from build123d import *

# Parameters (mm, degrees)
F0_R     = 1.75
F0_R_2   = 1.981
F0_W     = 100
F0_H     = 7.5
F1_DEPTH = 7.5


with BuildPart() as f1:
    # F0 (on Top) → F1 (new body)
    with BuildSketch(Plane.XY):
        with BuildLine():
            Line((109.467205, 397.377165), (-77.832795, 397.377165))
            ThreePointArc((-77.832795, 397.377165), (-82.322924, 395.517293), (-84.182795, 391.027165))
            Line((-84.182795, 391.027165), (-84.182795, 374.177175))
            Line((-84.182795, 374.177175), (-76.682795, 374.177175))
            Line((-76.682795, 374.177175), (-76.682795, 366.677175))
            Line((-76.682795, 366.677175), (-84.182795, 366.677175))
            Line((-84.182795, 366.677175), (-84.182795, 324.227175))
            Line((-84.182795, 324.227175), (-76.682795, 324.227175))
            Line((-76.682795, 324.227175), (-76.682795, 316.727175))
            Line((-76.682795, 316.727175), (-84.182795, 316.727175))
            Line((-84.182795, 316.727175), (-84.182795, 274.277175))
            Line((-84.182795, 274.277175), (-76.682795, 274.277175))
            Line((-76.682795, 274.277175), (-76.682795, 266.777175))
            Line((-76.682795, 266.777175), (-84.182795, 266.777175))
            Line((-84.182795, 266.777175), (-84.182795, 224.327175))
            Line((-84.182795, 224.327175), (-76.682795, 224.327175))
            Line((-76.682795, 224.327175), (-76.682795, 216.827175))
            Line((-76.682795, 216.827175), (-84.182795, 216.827175))
            Line((-84.182795, 216.827175), (-84.182795, 174.377175))
            Line((-84.182795, 174.377175), (-76.682795, 174.377175))
            Line((-76.682795, 174.377175), (-76.682795, 166.877175))
            Line((-76.682795, 166.877175), (-84.182795, 166.877175))
            Line((-84.182795, 166.877175), (-84.182795, 124.427175))
            Line((-84.182795, 124.427175), (-76.682795, 124.427175))
            Line((-76.682795, 124.427175), (-76.682795, 116.927175))
            Line((-76.682795, 116.927175), (-84.182795, 116.927175))
            Line((-84.182795, 116.927175), (-84.182795, 74.477175))
            Line((-84.182795, 74.477175), (-76.682795, 74.477175))
            Line((-76.682795, 74.477175), (-76.682795, 66.977175))
            Line((-76.682795, 66.977175), (-84.182795, 66.977175))
            Line((-84.182795, 66.977175), (-84.182795, 24.527175))
            Line((-84.182795, 24.527175), (-76.682795, 24.527175))
            Line((-76.682795, 24.527175), (-76.682795, 17.027175))
            Line((-76.682795, 17.027175), (-84.182795, 17.027175))
            Line((-84.182795, 17.027175), (-84.182795, -25.422825))
            Line((-84.182795, -25.422825), (-76.682795, -25.422825))
            Line((-76.682795, -25.422825), (-76.682795, -32.922825))
            Line((-76.682795, -32.922825), (-84.182795, -32.922825))
            Line((-84.182795, -32.922825), (-84.182795, -75.372825))
            Line((-84.182795, -75.372825), (-76.682795, -75.372825))
            Line((-76.682795, -75.372825), (-76.682795, -82.872825))
            Line((-76.682795, -82.872825), (-84.182795, -82.872825))
            Line((-84.182795, -82.872825), (-84.182795, -125.322825))
            Line((-84.182795, -125.322825), (-76.682795, -125.322825))
            Line((-76.682795, -125.322825), (-76.682795, -132.822825))
            Line((-76.682795, -132.822825), (-84.182795, -132.822825))
            Line((-84.182795, -132.822825), (-84.182795, -175.272825))
            Line((-84.182795, -175.272825), (-76.682795, -175.272825))
            Line((-76.682795, -175.272825), (-76.682795, -182.772825))
            Line((-76.682795, -182.772825), (-84.182795, -182.772825))
            Line((-84.182795, -182.772825), (-84.182795, -225.222825))
            Line((-84.182795, -225.222825), (-76.682795, -225.222825))
            Line((-76.682795, -225.222825), (-76.682795, -232.722825))
            Line((-76.682795, -232.722825), (-84.182795, -232.722825))
            Line((-84.182795, -232.722825), (-84.182795, -275.172825))
            Line((-84.182795, -275.172825), (-76.682795, -275.172825))
            Line((-76.682795, -275.172825), (-76.682795, -282.672825))
            Line((-76.682795, -282.672825), (-84.182795, -282.672825))
            Line((-84.182795, -282.672825), (-84.182795, -325.122825))
            Line((-84.182795, -325.122825), (-76.682795, -325.122825))
            Line((-76.682795, -325.122825), (-76.682795, -332.622825))
            Line((-76.682795, -332.622825), (-84.182795, -332.622825))
            Line((-84.182795, -332.622825), (-84.182795, -346.272835))
            ThreePointArc((-84.182795, -346.272835), (-82.322924, -350.762964), (-77.832795, -352.622835))
            Line((-77.832795, -352.622835), (109.467205, -352.622835))
            ThreePointArc((109.467205, -352.622835), (113.957333, -350.762964), (115.817205, -346.272835))
            Line((115.817205, -346.272835), (115.817205, -332.622835))
            Line((115.817205, -332.622835), (108.317205, -332.622835))
            Line((108.317205, -332.622835), (108.317205, -325.122835))
            Line((108.317205, -325.122835), (115.817205, -325.122835))
            Line((115.817205, -325.122835), (115.817205, -282.672835))
            Line((115.817205, -282.672835), (108.317205, -282.672835))
            Line((108.317205, -282.672835), (108.317205, -275.172835))
            Line((108.317205, -275.172835), (115.817205, -275.172835))
            Line((115.817205, -275.172835), (115.817205, -232.722835))
            Line((115.817205, -232.722835), (108.317205, -232.722835))
            Line((108.317205, -232.722835), (108.317205, -225.222835))
            Line((108.317205, -225.222835), (115.817205, -225.222835))
            Line((115.817205, -225.222835), (115.817205, -182.772835))
            Line((115.817205, -182.772835), (108.317205, -182.772835))
            Line((108.317205, -182.772835), (108.317205, -175.272835))
            Line((108.317205, -175.272835), (115.817205, -175.272835))
            Line((115.817205, -175.272835), (115.817205, -132.822835))
            Line((115.817205, -132.822835), (108.317205, -132.822835))
            Line((108.317205, -132.822835), (108.317205, -125.322835))
            Line((108.317205, -125.322835), (115.817205, -125.322835))
            Line((115.817205, -125.322835), (115.817205, -82.872835))
            Line((115.817205, -82.872835), (108.317205, -82.872835))
            Line((108.317205, -82.872835), (108.317205, -75.372835))
            Line((108.317205, -75.372835), (115.817205, -75.372835))
            Line((115.817205, -75.372835), (115.817205, -32.922835))
            Line((115.817205, -32.922835), (108.317205, -32.922835))
            Line((108.317205, -32.922835), (108.317205, -25.422835))
            Line((108.317205, -25.422835), (115.817205, -25.422835))
            Line((115.817205, -25.422835), (115.817205, 17.027165))
            Line((115.817205, 17.027165), (108.317205, 17.027165))
            Line((108.317205, 17.027165), (108.317205, 24.527165))
            Line((108.317205, 24.527165), (115.817205, 24.527165))
            Line((115.817205, 24.527165), (115.817205, 66.977165))
            Line((115.817205, 66.977165), (108.317205, 66.977165))
            Line((108.317205, 66.977165), (108.317205, 74.477165))
            Line((108.317205, 74.477165), (115.817205, 74.477165))
            Line((115.817205, 74.477165), (115.817205, 116.927165))
            Line((115.817205, 116.927165), (108.317205, 116.927165))
            Line((108.317205, 116.927165), (108.317205, 124.427165))
            Line((108.317205, 124.427165), (115.817205, 124.427165))
            Line((115.817205, 124.427165), (115.817205, 166.877165))
            Line((115.817205, 166.877165), (108.317205, 166.877165))
            Line((108.317205, 166.877165), (108.317205, 174.377165))
            Line((108.317205, 174.377165), (115.817205, 174.377165))
            Line((115.817205, 174.377165), (115.817205, 216.827165))
            Line((115.817205, 216.827165), (108.317205, 216.827165))
            Line((108.317205, 216.827165), (108.317205, 224.327165))
            Line((108.317205, 224.327165), (115.817205, 224.327165))
            Line((115.817205, 224.327165), (115.817205, 266.777165))
            Line((115.817205, 266.777165), (108.317205, 266.777165))
            Line((108.317205, 266.777165), (108.317205, 274.277165))
            Line((108.317205, 274.277165), (115.817205, 274.277165))
            Line((115.817205, 274.277165), (115.817205, 316.727165))
            Line((115.817205, 316.727165), (108.317205, 316.727165))
            Line((108.317205, 316.727165), (108.317205, 324.227165))
            Line((108.317205, 324.227165), (115.817205, 324.227165))
            Line((115.817205, 324.227165), (115.817205, 366.677165))
            Line((115.817205, 366.677165), (108.317205, 366.677165))
            Line((108.317205, 366.677165), (108.317205, 374.177165))
            Line((108.317205, 374.177165), (115.817205, 374.177165))
            Line((115.817205, 374.177165), (115.817205, 391.027165))
            ThreePointArc((115.817205, 391.027165), (113.957333, 395.517293), (109.467205, 397.377165))
        make_face()
        with Locations((-59.182573, -285.634338)):
            Circle(F0_R, mode=Mode.SUBTRACT)
        Polygon((-48.162773, -168.857838), (-41.787373, -168.857838), (-29.747773, -168.857838), (-23.372373, -168.857838), (-17.352573, -168.857838), (-17.352573, -180.237038), (-17.352573, -282.395838), (-14.177573, -282.395838), (-14.177573, -284.935838), (-14.177573, -286.586838), (-14.177573, -288.009238), (-13.177573, -288.009238), (-13.177573, -288.872838), (-13.177573, -289.372838), (-14.177573, -289.372838), (-32.592573, -289.372838), (-33.227573, -289.372838), (-51.642573, -289.372838), (-52.642573, -289.372838), (-52.642573, -288.872838), (-54.182573, -288.872838), (-54.182573, -282.395838), (-54.182573, -180.237038), (-54.182573, -168.857838), align=None, mode=Mode.SUBTRACT)
        with Locations((-59.182573, -135.202538)):
            Circle(F0_R_2, mode=Mode.SUBTRACT)
        Polygon((-52.642573, -138.872838), (-52.642573, -138.009238), (-54.182573, -138.009238), (-54.182573, -132.395838), (-54.182573, -30.237038), (-54.182573, -18.857838), (-48.162773, -18.857838), (-41.787373, -18.857838), (-29.747773, -18.857838), (-23.372373, -18.857838), (-17.352573, -18.857838), (-17.352573, -30.237038), (-17.352573, -132.395838), (-14.177573, -132.395838), (-14.177573, -134.935838), (-14.177573, -136.586838), (-14.177573, -138.009238), (-13.177573, -138.009238), (-13.177573, -138.872838), (-13.177573, -139.372838), (-14.177573, -139.372838), (-32.592573, -139.372838), (-33.227573, -139.372838), (-51.642573, -139.372838), (-52.642573, -139.372838), align=None, mode=Mode.SUBTRACT)
        with Locations((15.817205, -342.622835)):
            Rectangle(F0_W, F0_H, mode=Mode.SUBTRACT)
        with Locations((40.822427, -285.634338)):
            Circle(F0_R, mode=Mode.SUBTRACT)
        Polygon((-4.182573, -288.872838), (-4.182573, -282.395838), (-4.182573, -180.237038), (-4.182573, -168.857838), (1.837227, -168.857838), (8.212627, -168.857838), (20.252227, -168.857838), (26.627627, -168.857838), (32.647427, -168.857838), (32.647427, -180.237038), (32.647427, -282.395838), (35.822427, -282.395838), (35.822427, -284.935838), (35.822427, -286.586838), (35.822427, -288.009238), (36.822427, -288.009238), (36.822427, -288.872838), (36.822427, -289.372838), (35.822427, -289.372838), (16.772427, -289.372838), (-1.642573, -289.372838), (-2.642573, -289.372838), (-2.642573, -288.872838), align=None, mode=Mode.SUBTRACT)
        Polygon((32.647427, -18.857838), (32.647427, -30.237038), (32.647427, -132.395838), (35.822427, -132.395838), (35.822427, -134.935838), (35.822427, -136.586838), (35.822427, -138.009238), (36.822427, -138.009238), (36.822427, -138.872838), (36.822427, -139.372838), (35.822427, -139.372838), (17.407427, -139.372838), (16.772427, -139.372838), (-1.642573, -139.372838), (-2.642573, -139.372838), (-2.642573, -138.872838), (-2.642573, -138.009238), (-4.182573, -138.009238), (-4.182573, -132.395838), (-4.182573, -30.237038), (-4.182573, -18.857838), (1.837227, -18.857838), (8.212627, -18.857838), (20.252227, -18.857838), (26.627627, -18.857838), align=None, mode=Mode.SUBTRACT)
        with Locations((40.822427, -135.202538)):
            Circle(F0_R_2, mode=Mode.SUBTRACT)
        with Locations((15.817205, 387.377165)):
            Rectangle(F0_W, F0_H, mode=Mode.SUBTRACT)
    extrude(amount=F1_DEPTH)


solid = f1.part
The model under review builds one solid part; all positions refer to its coordinate system, in mm. Round coordinates to 2 decimals unless told otherwise and drop trailing zeros. Loops run counter-clockwise (first coordinate to the right, second up) from the corner with the lowest first, then second, coordinate; pieces in that order, holes last. Notation, with made-up numbers: M 46.5,78 L 69.5,78 A26 ccw 69.5,106 Z; hole C -7.75,-29.75 d6. An arc over 180 degrees is marked long. Answer as CSV lines item,"result". Start each with the question number.
Item 1: Insertion check: P1, Ø3, axis at x = 30, y = 301, coming from the -Z side; P2, Ø2, axis at x = 111, z = 5.5, coming from the -Y side; P3, Ø2, axis at x = -79, z = 3.5, coming from the +Y side; P4, Ø4, axis at y = -127.5, z = 3, coming from the +X side. Each pin has a flat end and moves straight along its axis. Give the tip position at first contact, or say it passes through.
Item 2: Consider section C-C (z = 3.75). State how many separate pieces and enclosed holes the cut face has, then the cut area to 3 significant figures.
Item 3: Consider section A-A (x = 17.5). Write out the cut boundary in (y, z), then the cut area to 3 significant figures.
Item 4: Consider section B-B (y = -103). Write out the cut boundary in (x, z).
Item 5: Wall thickness on line 1 (Y direction, x = 20.5, z = 5.25); line 2 (Y direction, x = 45, z = 6.5); line 3 (X direction, y = -204, z = 1.5): over which ranges is each line inside the solid? List them lowest first. Write a range as [from, to].
Answer:
1,P1,"stops at z = 0"
1,P2,"stops at y = -352.6"
1,P3,"stops at y = 397.37"
1,P4,"stops at x = 108.32"
2,separate pieces,"1"
2,enclosed holes,"10"
2,area,"129,000 mm^2"
3,outline,"M -352.62,0 L -346.37,0 L -346.37,7.5 L -352.62,7.5 Z; M -338.87,0 L -289.37,0 L -289.37,7.5 L -338.87,7.5 Z; M -168.86,0 L -139.37,0 L -139.37,7.5 L -168.86,7.5 Z; M -18.86,0 L 383.63,0 L 383.63,7.5 L -18.86,7.5 Z; M 391.13,0 L 397.38,0 L 397.38,7.5 L 391.13,7.5 Z"
3,area,"3,700 mm^2"
4,outline,"M -84.18,0 L -54.18,0 L -54.18,7.5 L -84.18,7.5 Z; M -17.35,0 L -4.18,0 L -4.18,7.5 L -17.35,7.5 Z; M 32.65,0 L 115.82,0 L 115.82,7.5 L 32.65,7.5 Z"
5,line 1,"y = [-352.62, -346.37], [-338.87, -289.37], [-168.86, -139.37], [-18.86, 383.63], [391.13, 397.38]"
5,line 2,"y = [-352.62, -346.37], [-338.87, 383.63], [391.13, 397.38]"
5,line 3,"x = [-84.18, -54.18], [-17.35, -4.18], [32.65, 115.82]"
